Model file for the job. Use its own axes, mm. Give positions to 0.01 mm unless a question says otherwise; leave off trailing zeros. Write each loop counter-clockwise with the first axis right and the second up, starting at its lowest first coordinate (ties: lowest second). Pieces come first, ordered by that corner, then holes. Notation, with made-up numbers: (62.25, 9.5) - (77.25, 9.5) arc R20 ccw to (77.25, 29.5) - close; hole circle Ø1 at (67.25, 72). An arc over 180 degrees is marked (long way). Use a Markdown table: item, result. Add a question column.
```python
from build123d import *

# Parameters (mm, degrees)
SKETCH1_R           = 15.875
BOSS_EXTRUDE1_DEPTH = 609.6
SKETCH2_R           = 2.1971
CUT_EXTRUDE1_DEPTH  = 76.2


with BuildPart() as part:
    # Sketch1 → Boss-Extrude1 (new body)
    with BuildSketch(Plane(origin=(0, 0, 0), x_dir=(1, 0, 0), z_dir=(0, 1, 0))):
        with Locations(Location((0, 0, 0), (0, 0, 90))):
            Circle(SKETCH1_R)
    extrude(amount=BOSS_EXTRUDE1_DEPTH)

    # Sketch2 → Cut-Extrude1 (cut)
    with BuildSketch(Plane.XZ):
        with Locations(Location((0, 11.43, 0), (0, 0, 270))):
            Circle(SKETCH2_R)
        with Locations(Location((11.43, 0, 0), (0, 0, 270))):
            Circle(SKETCH2_R)
        with Locations(Location((0, -11.43, 0), (0, 0, 270))):
            Circle(SKETCH2_R)
        with Locations(Location((-11.43, 0, 0), (0, 0, 270))):
            Circle(SKETCH2_R)
    extrude(amount=-CUT_EXTRUDE1_DEPTH, mode=Mode.SUBTRACT)


solid = part.part
```
(1) Band-saw the part on A-A (y = 330.5). Write the cut outline in (x, z) (3 decimals), then the cut area to 3 significant figures.
(2) Flat gauge pins, fed straight in: pin 1 (2 mm diameter, centred on x = -5.5, y = 274, fed in from +Z); pin 2 (4 mm diameter, centred on x = 0, z = 11.43, fed in from -Y); pin 3 (8 mm diameter, centred on x = 6, y = 401.5, fed in from -Z). Where does each tip first touch, or does it go through?
(3) Probe probe 1 along X at (y, z) = (41, 0) (3 decimals); probe 2 along Z at (x, y) = (-1.5, 511); probe 3 along X at (y, z) = (75, -11). List the from-to ranges inside material, lowest first. Write a range as [from, to].
Model answer:
| question | item | result |
|---|---|---|
| 1 | outline | circle Ø31.75 at (0, 0) |
| 1 | area | 792 mm^2 |
| 2 | pin 1 | stops at z = 15.22 |
| 2 | pin 2 | stops at y = 76.2 |
| 2 | pin 3 | stops at z = -15.75 |
| 3 | probe 1 | x = [-15.875, -13.627], [-9.233, 9.233], [13.627, 15.875] |
| 3 | probe 2 | z = [-15.8, 15.8] |
| 3 | probe 3 | x = [-11.45, -2.15], [2.15, 11.45] |
